from build123d import *

# Parameters (mm, degrees)
F0_W     = 1112
F0_H     = 496
F1_DEPTH = 176
F2_W     = 1101
F2_H     = 336
F3_DEPTH = 20
F4_W     = 1011
F4_H     = 246
F5_DEPTH = 15


with BuildPart() as f1:
    # F0 (on Front) → F1 (new body)
    with BuildSketch(Plane.XZ):
        Rectangle(F0_W, F0_H)
    extrude(amount=F1_DEPTH)

    # F2 (on face) → F3 (join)
    with BuildSketch(Plane.XZ.offset(176)):
        with Locations((0, -55.5)):
            Rectangle(F2_W, F2_H)
    extrude(amount=F3_DEPTH)

    # F4 (on face) → F5 (cut)
    with BuildSketch(Plane.XZ.offset(196)):
        with Locations((0, -55.5)):
            Rectangle(F4_W, F4_H)
    extrude(amount=-F5_DEPTH, mode=Mode.SUBTRACT)


solid = f1.part
Geometry: final body of the model. Coordinates: model frame, mm. A direction names the side the tool comes from. Round coordinates to 2 decimals unless told otherwise and drop trailing zeros. Loops run counter-clockwise (first coordinate to the right, second up) from the corner with the lowest first, then second, coordinate; pieces in that order, holes last.
Q1. Section C-C on z = 147.5. Return loops of the section in (x, y).
Q2. Pin query (flat end, axial travel): P1, Ø6, axis at x = -147.5, y = -184, coming from the +Z side; P2, Ø6, axis at y = -190, z = -72.5, coming from the +X side; P3, Ø4.5, axis at y = -189.5, z = -18.5, coming from the -X side. Return the tip coordinate at first contact, or that it passes through.
Q3. Pull-direction query (X, two-part tool) for faces 5 (the flat face through (-8, -186, 112.5)), 6 (the flat face through (-7, -181, -54)), 7 (the flat face through (-556, -87, -3)), 8 (the flat face through (556, -87, -3)); classes: released by +X, released by -X, zero draft, split by the parting line, or undercut.
Q4. Access query for faces 1 (the flat face through (-550.5, -186, -58)), 2 (the flat face through (-8, -186, -223.5)), 3 (the flat face through (550.5, -186, -58)), 4 (the flat face through (-8, 0, 3)). Directions: +Z, -Z, +X, -X, +Y, -Y. A direction counts if a zero-diameter tool reaches every point of the face in a straight line with its end or side. Return the directions, or none.
Q5. Section B-B on x = 60.5. Return loops of the section in (y, z).
Q6. Material intervals for L1, parallel to X at y = -184, z = -68; L2, parallel to Y at x = -165.5, z = 48; L3, parallel to Y at x = 288, z = 143, sorted ascending.
Q7. Section A-A on z = -38.5. Return loops of the section in (x, y).
Evaluation:
1. outline: (-556, -176) - (556, -176) - (556, 0) - (-556, 0) - close
2. P1: stops at z = 112.5
2. P2: stops at x = 550.5
2. P3: stops at x = -550.5
3. face 5: zero draft
3. face 6: undercut
3. face 7: released by -X
3. face 8: released by +X
4. face 1: +Z, -Z, -X, -Y
4. face 2: -Z, +X, -X, -Y
4. face 3: +Z, -Z, +X, -Y
4. face 4: +Z, -Z, +X, -X, +Y
5. outline: (-196, -223.5) - (-176, -223.5) - (-176, -248) - (0, -248) - (0, 248) - (-176, 248) - (-176, 112.5) - (-196, 112.5) - (-196, 67.5) - (-181, 67.5) - (-181, -178.5) - (-196, -178.5) - close
6. L1: x = -550.5 to -505.5, 505.5 to 550.5
6. L2: y = -181 to 0
6. L3: y = -176 to 0
7. outline: (-556, -176) - (-550.5, -176) - (-550.5, -196) - (-505.5, -196) - (-505.5, -181) - (505.5, -181) - (505.5, -196) - (550.5, -196) - (550.5, -176) - (556, -176) - (556, 0) - (-556, 0) - close
